from build123d import *

# Parameters (mm, degrees)
BOSS_EXTRUDE1_DEPTH = 2
SKETCH2_R           = 3
CUT_EXTRUDE1_DEPTH  = 5
CHAMFER1_SIZE       = 3


with BuildPart() as part:
    # Sketch1 → Boss-Extrude1 (new body, symmetric)
    with BuildSketch(Plane.XY):
        Polygon((-20, -30), (-20, 30), (0, 30), (20, -10), (20, -30), align=None)
    extrude(amount=BOSS_EXTRUDE1_DEPTH, both=True)

    # Sketch2 → Cut-Extrude1 (cut, through all)
    with BuildSketch(Plane.XY.offset(2)):
        with Locations((-10, 20)):
            Circle(SKETCH2_R)
        with Locations((-10, -20)):
            Circle(SKETCH2_R)
        with Locations((10, -20)):
            Circle(SKETCH2_R)
    extrude(amount=-CUT_EXTRUDE1_DEPTH, mode=Mode.SUBTRACT)

    # Chamfer1
    chamfer1_edges = [part.edges().sort_by_distance(p)[0] for p in [
        (-13, 20, 2),
        (-13, -20, 2),
        (7, -20, 2),
    ]]
    chamfer(chamfer1_edges, length=CHAMFER1_SIZE)


solid = part.part
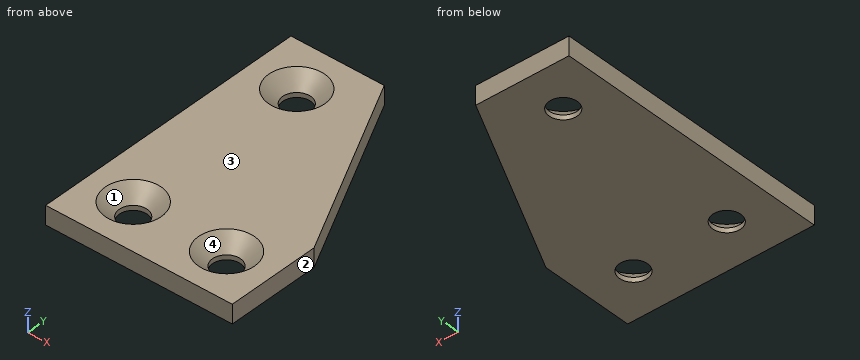
Geometry: final body of the model. Coordinates: model frame, mm. Face numbers are marked on the shaded views. Give positions to 0.01 mm unless a question says otherwise; leave off trailing zeros. Loops run counter-clockwise (first coordinate to the right, second up) from the corner with the lowest first, then second, coordinate; pieces in that order, holes last. Notation, with made-up numbers: M -24,85 L 19,85 A20 cw 19,117 Z; hole C 23.25,-27 d9. An arc over 180 degrees is marked long. Put each result on its own line as item: value.
1) Material intervals for L1, parallel to Y at x = -10, z = -1.6; L2, parallel to X at y = -18, z = 1.3; L3, parallel to Y at x = -8, z = 1.55, sorted ascending. Write a range as from..to.
Computed values:
L1: y = -30..-23, -17..17, 23..30
L2: x = -20..-14.91, -5.09..5.09, 14.91..20
L3: y = -30..-25.18, -14.82..14.82, 25.18..30
2) Mould query, pull axis X, two halves, no side actions, for the marked faces 1, 2, 3 and 4. Classes: released by +X, released by -X, zero draft, split by the parting line, or undercut.
Computed values:
face 1: undercut
face 2: released by +X
face 3: zero draft
face 4: undercut
3) Cut plane A-A, the plane y = -20. Return the cut outline in (x, z).
Computed values:
outline: M -20,-2 L -13,-2 L -13,-1 L -16,2 L -20,2 Z; M -7,-2 L 7,-2 L 7,-1 L 4,2 L -4,2 L -7,-1 Z; M 13,-2 L 20,-2 L 20,2 L 16,2 L 13,-1 Z
4) Cut plane D-D, the plane y = 20. Return the cut outline in (x, z).
Computed values:
outline: M -20,-2 L -13,-2 L -13,-1 L -16,2 L -20,2 Z; M -7,-2 L 5,-2 L 5,2 L -4,2 L -7,-1 Z
5) Cut plane C-C, the plane z = 0.6. Return the cut outline in (x, y).
Computed values:
outline: M -20,-30 L 20,-30 L 20,-10 L 0,30 L -20,30 Z; hole C -10,-20 d9.2; hole C -10,20 d9.2; hole C 10,-20 d9.2
6) First-contact query: P1, Ø5.5, axis at x = 10, y = -20, coming from the +Z side; P2, Ø9.5, axis at x = -10, y = -20, coming from the +Z side; P3, Ø2, axis at x = 8, z = -0.5, coming from the +Y side. Flat tips, straight axial feed; report the tip coordinate or a pass-through.
Computed values:
P1: passes through
P2: stops at z = 0.75
P3: stops at y = 16
7) Cut plane B-B, the plane x = 10. Return the cut outline in (y, z).
Computed values:
outline: M -30,-2 L -23,-2 L -23,-1 L -26,2 L -30,2 Z; M -17,-2 L 10,-2 L 10,2 L -14,2 L -17,-1 Z
